Design review of the part built by this model. Coordinates are the model's own, in mm. Round coordinates to 2 decimals unless told otherwise and drop trailing zeros. Write each loop counter-clockwise with the first axis right and the second up, starting at its lowest first coordinate (ties: lowest second). Pieces come first, ordered by that corner, then holes.
from build123d import *

# Parameters (mm, degrees)
SKETCH2_R           = 1.7
BOSS_EXTRUDE1_DEPTH = 5


with BuildPart() as part:
    # Sketch2 → Boss-Extrude1 (new body)
    with BuildSketch(Plane.XY.offset(0.022274507)):
        with BuildLine():
            Line((26.815853016, -16.790117538), (20.584977895, -15.389970557))
            Line((20.584977895, -15.389970557), (20.584977895, 15.389970557))
            Line((20.584977895, 15.389970557), (26.298427654, 16.636497968))
            ThreePointArc((26.298427654, 16.636497968), (27.556656853, 16.885073389), (28.828845221, 16.722385915))
            Line((28.828845221, 16.722385915), (34.799540996, 15.389970557))
            Line((34.799540996, 15.389970557), (34.799540996, 10.589698359))
            ThreePointArc((34.799540996, 10.589698359), (30.183127704, 0.060029443), (34.799540996, -10.469639472))
            Line((34.799540996, -10.469639472), (34.799540996, -15.389970557))
            Line((34.799540996, -15.389970557), (28.568665876, -16.790117538))
            ThreePointArc((28.568665876, -16.790117538), (27.692259446, -16.887374052), (26.815853016, -16.790117538))
        make_face()
        with Locations((27.692259446, -12.889970557)):
            Circle(SKETCH2_R, mode=Mode.SUBTRACT)
        with Locations((27.692259446, 12.889970557)):
            Circle(SKETCH2_R, mode=Mode.SUBTRACT)
    extrude(amount=BOSS_EXTRUDE1_DEPTH)


solid = part.part
1) Add section D-D on x = 23.5. State the section outline as (y, z) points (3 decimals), and give its area (3 significant figures).
2) Add section A-A on y = -12.5. State the section outline as (x, z) points, and give its area (3 significant figures).
3) Add section C-C on z = 0.4. State the section outline as (x, y) points.
4) Add section B-B on x = 33.75. State the section outline as (y, z) points.
5) For P1, Ø5.5, axis at x = 27.69, y = -12.89, coming from the +Z side; P2, Ø1, axis at y = 3, z = 4, coming from the +X side; P3, Ø1, axis at y = 9.5, z = 1.5, coming from the +X side; P4, Ø1, axis at x = 32, z = 3.5, coming from the +Y side, all flat-tipped, find the tip position at first contact; note any pin that passes through.
6) For line 1 along Y through (x, z) = (28.25, 1.4); line 2 along Y through (x, z) = (27.25, 0.6); line 3 along Y through (x, z) = (33.5, 0.3), list the stretches that pass through material, from the lowest coordinate up.
7) The part is to be moulded in two halves that separate along Z. For faces 1 (the face through (26, 0, 5.022)), 2 (the face through (26, 0, 0.022)), 3 (the face through (34.8, -13, 2)), say which applies: pulls with the +Z half, pulls with the -Z half, needs draft (parallel to the pull), parting line crosses it, or undercut.
Computed:
1. outline: (-16.045, 0.022) - (16.026, 0.022) - (16.026, 5.022) - (-16.045, 5.022) - close
1. area: 160 mm2
2. outline: (20.58, 0.02) - (26.04, 0.02) - (26.04, 5.02) - (20.58, 5.02) - close; (29.35, 0.02) - (34.8, 0.02) - (34.8, 5.02) - (29.35, 5.02) - close
2. area: 54.5 mm2
3. outline: (20.58, -15.39) - (26.82, -16.79) arc R4 ccw to (28.57, -16.79) - (34.8, -15.39) - (34.8, -10.47) arc R14.32 cw to (34.8, 10.59) - (34.8, 15.39) - (28.83, 16.72) arc R4 ccw to (26.3, 16.64) - (20.58, 15.39) - close; hole circle Ø3.4 at (27.69, -12.89); hole circle Ø3.4 at (27.69, 12.89)
4. outline: (-15.63, 0.02) - (-9.4, 0.02) - (-9.4, 5.02) - (-15.63, 5.02) - close; (9.52, 0.02) - (15.62, 0.02) - (15.62, 5.02) - (9.52, 5.02) - close
5. P1: stops at z = 5.02
5. P2: stops at x = 30.6
5. P3: stops at x = 34.2
5. P4: stops at y = 16.13
6. line 1: y = -16.85 to -14.5, -11.28 to 11.28, 14.5 to 16.85
6. line 2: y = -16.86 to -14.53, -11.25 to 11.25, 14.53 to 16.86
6. line 3: y = -15.68 to -9.1, 9.22 to 15.68
7. face 1: pulls with the +Z half
7. face 2: pulls with the -Z half
7. face 3: needs draft
